from build123d import *

# Parameters (mm, degrees)
F1_DEPTH    = 63.5
F2_T        = -2.54
F4_DEPTH    = 25.4
F1_FACE_R   = 3.81
F1_FACE_R_2 = 3.814678
F5_DEPTH    = 9.652
F7_R        = 3.80479
F8_DEPTH    = 90.678
F9_DEPTH    = 0.254
F7_R_2      = 3.81
F10_DEPTH   = 90.424
F11_R       = 3.910877
F12_DEPTH   = 0.254


with BuildPart() as f1:
    # F0 (on Top) → F1 (new body)
    with BuildSketch(Plane.XY):
        Polygon((76.681964, 0), (0, 38.1), (0, 0), (0, -38.1), align=None)
        Polygon((0, 0), (0, 38.1), (-88.9, 31.75), (-88.9, 0), align=None)
        Polygon((0, -38.1), (0, 0), (-88.9, 0), (-88.9, -31.75), align=None)
    extrude(amount=F1_DEPTH)

    # F2
    f2_openings = [f1.faces().sort_by_distance(p)[0] for p in [
        (-21.133783, 0, 63.5),
    ]]
    offset(amount=F2_T, openings=f2_openings)

    # F3 (on face) → F4 (cut)
    with BuildSketch(Plane(origin=(0, 0, 0), x_dir=(1, 0, 0), z_dir=(0, 0, -1))):
        with BuildLine():
            ThreePointArc((3.814678, -4.445), (2.697385, -1.747615), (0, -0.630322))
            ThreePointArc((0, -0.630322), (-2.697385, -7.142385), (3.814678, -4.445))
        make_face()
        with BuildLine():
            ThreePointArc((3.81, 4.445), (-2.694077, 7.139077), (0, 0.635))
            ThreePointArc((0, 0.635), (2.694077, 1.750923), (3.81, 4.445))
        make_face()
    extrude(amount=-F4_DEPTH, mode=Mode.SUBTRACT)

    # F1_face (on face) → F5 (join)
    with BuildSketch(Plane(origin=(-21.133783, 0, 0), x_dir=(1, 0, 0), z_dir=(0, 0, -1))):
        Polygon((21.133783, -38.1), (97.815747, 0), (21.133783, 38.1), (-67.766217, 31.75), (-67.766217, -31.75), align=None)
        with Locations((21.133783, 4.445)):
            Circle(F1_FACE_R, mode=Mode.SUBTRACT)
        with Locations((21.133783, -4.445)):
            Circle(F1_FACE_R_2, mode=Mode.SUBTRACT)
    extrude(amount=F5_DEPTH)

    # F7 (on face) → F8 (cut)
    with BuildSketch(Plane(origin=(-88.9, 0, 0), x_dir=(0, -1, 0), z_dir=(-1, 0, 0))):
        with Locations((-4.496679, -4.826)):
            Circle(F7_R)
    extrude(amount=-F8_DEPTH, mode=Mode.SUBTRACT)

    # F6 (on face) → F9 (join)
    with BuildSketch(Plane(origin=(0, 0, -9.652), x_dir=(1, 0, 0), z_dir=(0, 0, -1))):
        with BuildLine():
            ThreePointArc((3.814678, -4.445), (0, -0.630322), (-3.814678, -4.445))
            ThreePointArc((-3.814678, -4.445), (0, -8.259678), (3.814678, -4.445))
        make_face()
    extrude(amount=-F9_DEPTH)

    # F7 (on face) → F10 (cut)
    with BuildSketch(Plane(origin=(-88.9, 0, 0), x_dir=(0, -1, 0), z_dir=(-1, 0, 0))):
        with Locations((4.593814, -4.826)):
            Circle(F7_R_2)
    extrude(amount=-F10_DEPTH, mode=Mode.SUBTRACT)

    # F11 (on face) → F12 (join)
    with BuildSketch(Plane(origin=(0, 0, -9.652), x_dir=(1, 0, 0), z_dir=(0, 0, -1))):
        with Locations((0, 4.445)):
            Circle(F11_R)
    extrude(amount=-F12_DEPTH)


solid = f1.part
Work out the finished part from the listing and answer in its coordinate system (mm). A direction names the side the tool comes from. Round coordinates to 2 decimals unless told otherwise and drop trailing zeros. Write each loop counter-clockwise with the first axis right and the second up, starting at its lowest first coordinate (ties: lowest second). Pieces come first, ordered by that corner, then holes. Notation, with made-up numbers: (73, -1) - (112, -1) arc R16 ccw to (112, 5) - close; hole circle Ø8 at (-37.75, -6). An arc over 180 degrees is marked (long way). Answer in a Markdown table with one row per item. Add a question column.
1. A cutting plane is placed at D-D, the plane y = 24.5. Determine the outline of the cut face in (x, z), and give its area (3 significant figures).
2. The mould has two halves that part along X. Classify faces 4 (the flat face through (-26, 0, 2.54)), 5 (the flat face through (37.8, 19.32, 27.44)), 6 (the flat face through (-43.83, -34.97, 27.44)), 7 (the flat face through (-42.834, 32.494, 32.593)): +X half, -X half, draft (parallel to the pull), parting line (faces both ways), or undercut.
3. Find the intervals of material crossed by line 1 along Y through (x, z) = (0, -3) (3 decimals); line 2 along Z through (x, y) = (-39.5, 10.5); line 3 along Y through (x, z) = (39, 58.5), in increasing order. Write a range as from..to.
4. A cutting plane is placed at A-A, the plane z = 5.5. Determine the outline of the cut face in (x, y).
5. For faces 1 (the flat face through (38.88, -18.78, 27.44)), 2 (the flat face through (34.73, -18.01, 32.59)), 3 (the cylindrical face through (-44.321, -0.787, -4.658)), determine the directions among +Z, -Z, +X, -X, +Y, -Y from which every point of the face is accessible in a straight line to the end or side of a thin tool.
6. A cutting plane is placed at B-B, the plane x = -14. Determine the outline of the cut face in (y, z), and give its area (3 significant figures).
7. A cutting plane is placed at C-C, the plane x = 50.5. Determine the outline of the cut face in (y, z).
8. Given pin 1 (21.5 mm diameter, centred on x = 30, y = 3.5, fed in from +Z); pin 2 (0.5 mm diameter, centred on y = -8, z = -4, fed in from -X); pin 3 (1 mm diameter, centred on x = -34, z = 7.5, fed in from -Y), each flat-ended and moving along its own axis, determine where each tip first touches the part or whether it passes through.
Worked out:
| question | item | result |
|---|---|---|
| 1 | outline | (-88.9, -9.65) - (27.37, -9.65) - (27.37, 63.5) - (21.66, 63.5) - (21.66, 2.54) - (-86.36, 2.54) - (-86.36, 63.5) - (-88.9, 63.5) - close |
| 1 | area | 1,920 mm^2 |
| 2 | face 4 | undercut |
| 2 | face 5 | +X half |
| 2 | face 6 | -X half |
| 2 | face 7 | undercut |
| 3 | line 1 | -38.1..-8.255, -0.635..0.63, 8.26..38.1 |
| 3 | line 2 | -9.65..2.54 |
| 3 | line 3 | -18.72..-15.89, 15.89..18.72 |
| 4 | outline | (-88.9, -31.75) - (0, -38.1) - (76.68, 0) - (0, 38.1) - (-88.9, 31.75) - close; hole (-86.36, -29.38) - (-0.51, -35.52) - (70.97, 0) - (-0.51, 35.52) - (-86.36, 29.38) - close |
| 5 | face 1 | +Z, -Z, +X, -Y |
| 5 | face 2 | +Z |
| 5 | face 3 | -X |
| 6 | outline | (-37.1, -9.65) - (37.1, -9.65) - (37.1, 63.5) - (34.55, 63.5) - (34.55, 2.54) - (-34.55, 2.54) - (-34.55, 63.5) - (-37.1, 63.5) - close; hole circle Ø7.62 at (-4.59, -4.83); hole circle Ø7.61 at (4.5, -4.83) |
| 6 | area | 1,120 mm^2 |
| 7 | outline | (-13.01, -9.65) - (13.01, -9.65) - (13.01, 63.5) - (10.17, 63.5) - (10.17, 2.54) - (-10.17, 2.54) - (-10.17, 63.5) - (-13.01, 63.5) - close |
| 8 | pin 1 | z = 2.54 |
| 8 | pin 2 | x = 1.52 |
| 8 | pin 3 | y = -35.71 |
